from build123d import *

# Parameters (mm, degrees)
EXTRUDE_1_DEPTH     = 7.5
FILLET_1_R          = 3
FILLET_3_R          = 6
SKETCH_2_R          = 1.5
CUT_EXTRUDE_1_DEPTH = 10
SKETCH_5_R          = 4.5
EXTRUDE_2_DEPTH     = 15
SKETCH_4_R          = 1.5
CUT_EXTRUDE_3_DEPTH = 39.639358173
FILLET_2_R          = 6


with BuildPart() as part:
    # 草图1 → 凸台-拉伸1 (new, symmetric)
    with BuildSketch(Plane.XY):
        Polygon((-28, 5), (-28, 0), (-14, 0), (-14, 15), (0, 15), (0, 20), (-19, 20), (-19, 5), align=None)
        Polygon((0, 20), (0, 15), (14, 15), (14, 0), (28, 0), (28, 5), (19, 5), (19, 20), align=None)
    extrude(amount=EXTRUDE_1_DEPTH, both=True)

    # 圆角1
    fillet_1_edges = [part.edges().sort_by_distance(p)[0] for p in [
        (-19, 5, 0),
        (-19, 20, 0),
        (19, 20, 0),
        (19, 5, 0),
    ]]
    fillet(fillet_1_edges, radius=FILLET_1_R)

    # 圆角3
    fillet_3_edges = [part.edges().sort_by_distance(p)[0] for p in [
        (-14, 15, 0),
        (14, 15, 0),
    ]]
    fillet(fillet_3_edges, radius=FILLET_3_R)

    # 草图2 → 切除-拉伸1 (cut)
    with BuildSketch(Plane(origin=(0, 5, 0), x_dir=(1, 0, 0), z_dir=(0, 1, 0))):
        with Locations(Location((25, -4.5, 0), (0, 0, 180))):
            Circle(SKETCH_2_R)
        with Locations(Location((25, 4.5, 0), (0, 0, 180))):
            Circle(SKETCH_2_R)
    cut_extrude_1 = extrude(amount=-CUT_EXTRUDE_1_DEPTH, mode=Mode.SUBTRACT)

    # 草图5 → 凸台-拉伸2 (add)
    with BuildSketch(Plane.XY.offset(7.5)):
        with Locations((0, 17.5)):
            Circle(SKETCH_5_R)
    extrude(amount=-EXTRUDE_2_DEPTH)

    # 草图4 → 切除-拉伸3 (cut, through all)
    with BuildSketch(Plane.XY.offset(7.5)):
        with Locations((0, 17.5)):
            Circle(SKETCH_4_R)
    extrude(amount=-CUT_EXTRUDE_3_DEPTH, mode=Mode.SUBTRACT)

    # 镜向2: 切除-拉伸1 across plane
    add(cut_extrude_1.mirror(Plane(origin=(0, 0, 0), x_dir=(0, 0, 1), z_dir=(1, 0, 0))), mode=Mode.SUBTRACT)

    # 圆角2
    fillet_2_edges = [part.edges().sort_by_distance(p)[0] for p in [
        (-3.741657387, 15, 0),
        (-3.741657387, 20, 0),
        (3.741657387, 15, 0),
        (3.741657387, 20, 0),
    ]]
    fillet(fillet_2_edges, radius=FILLET_2_R)


solid = part.part
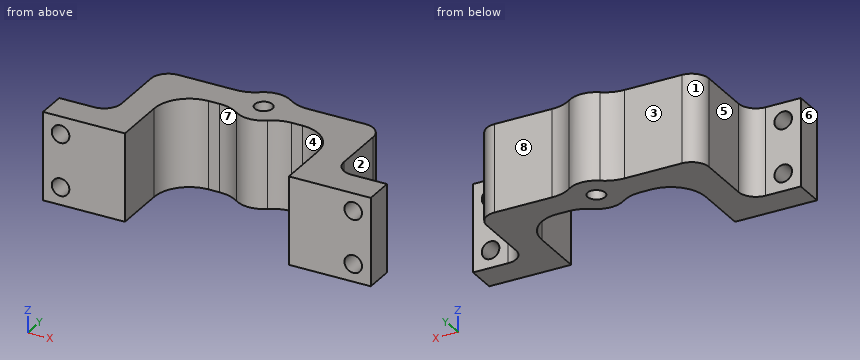
Could you check a few things on this model? Use its own coordinates, in mm. Face numbers are marked on the shaded views. A direction names the side the tool comes from. Give positions to 0.01 mm unless a question says otherwise; leave off trailing zeros. Write each loop counter-clockwise with the first axis right and the second up, starting at its lowest first coordinate (ties: lowest second). Pieces come first, ordered by that corner, then holes. Notation, with made-up numbers: (-19, 62) - (2, 62) arc R22 ccw to (2, 78) - close; hole circle Ø4 at (71.25, 81). An arc over 180 degrees is marked (long way). Use CSV: the item, a comma, the result in double quotes. Start each with the question number.
Item 1: I want a section at D-D, the plane z = 1.5. Please give me the cut outline in (x, y).
Item 2: If I drill on line 1 along Z through (x, y) = (-25, 1.75); line 2 along X through (y, z) = (2.75, -0.5); line 3 along X through (y, z) = (9, -3.75), over which ranges is the centre line in solid material (lowest first)?
Item 3: I want a section at C-C, the plane x = 0. Please give me the cut outline in (y, z), then the cut area to 3 significant figures.
Item 4: For the marked faces 5, 6, 7 and 8, which set-ups out of +Z, -Z, +X, -X, +Y, -Y let a thin tool reach every point of the face, with its end or its side?
Item 5: I'm going to push flat-ended pins straight in: pin 1 (2.5 mm diameter, centred on y = 12, z = -2.5, fed in from +X); pin 2 (0.6 mm diameter, centred on x = 7.5, z = -3.5, fed in from -Y); pin 3 (4 mm diameter, centred on x = -25, z = -4.5, fed in from -Y); pin 4 (6.5 mm diameter, centred on x = -26, z = -3.5, fed in from +Y). Where does each tip first touch, or does it pass through?
Item 6: I want a section at A-A, the plane y = 2.75. Please give me the cut outline in (x, z), then the cut area to 3 significant figures.
Item 7: If we mould it in two halves opening along X, with no side actions, what happens to the marked faces 1, 2, 3 and 4? For each: pulls with the +X half, pulls with the -X half, needs draft (parallel to the pull), parting line crosses it, or undercut.
Item 8: I want a section at B-B, the plane x = 25. Please give me the cut outline in (y, z), then the cut area to 3 significant figures.
Findings:
1,outline,"(-28, 0) - (-14, 0) - (-14, 9) arc R6 cw to (-8, 15) - (-6.16, 15) arc R6 cw to (-2.64, 13.86) arc R4.5 ccw to (2.64, 13.86) arc R6 cw to (6.16, 15) - (8, 15) arc R6 cw to (14, 9) - (14, 0) - (28, 0) - (28, 5) - (22, 5) arc R3 cw to (19, 8) - (19, 17) arc R3 ccw to (16, 20) - (6.16, 20) arc R6 cw to (2.64, 21.14) arc R4.5 ccw to (-2.64, 21.14) arc R6 cw to (-6.16, 20) - (-16, 20) arc R3 ccw to (-19, 17) - (-19, 8) arc R3 cw to (-22, 5) - (-28, 5) - close; hole circle Ø3 at (0, 17.5)"
2,line 1,"z = -7.5 to -6, -3 to 3, 6 to 7.5"
2,line 2,"x = -28 to -14, 14 to 28"
2,line 3,"x = -19 to -14, 14 to 19"
3,outline,"(13, -7.5) - (16, -7.5) - (16, 7.5) - (13, 7.5) - close; (19, -7.5) - (22, -7.5) - (22, 7.5) - (19, 7.5) - close"
3,area,"90.0 mm2"
4,face 5,"+Z, -Z, -X, +Y"
4,face 6,"+Z, -Z, -X, +Y, -Y"
4,face 7,"+Z, -Z, -Y"
4,face 8,"+Z, -Z, +X, +Y"
5,pin 1,"stops at x = 19"
5,pin 2,"stops at y = 15"
5,pin 3,"stops at y = 0"
5,pin 4,"stops at y = 5"
6,outline,"(-28, -7.5) - (-14, -7.5) - (-14, 7.5) - (-28, 7.5) - close; (14, -7.5) - (28, -7.5) - (28, 7.5) - (14, 7.5) - close; hole circle Ø3 at (-25, -4.5); hole circle Ø3 at (-25, 4.5); hole circle Ø3 at (25, -4.5); hole circle Ø3 at (25, 4.5)"
6,area,"392 mm2"
7,face 1,"pulls with the -X half"
7,face 2,"pulls with the +X half"
7,face 3,"needs draft"
7,face 4,"undercut"
8,outline,"(0, -7.5) - (5, -7.5) - (5, -6) - (0, -6) - close; (0, -3) - (5, -3) - (5, 3) - (0, 3) - close; (0, 6) - (5, 6) - (5, 7.5) - (0, 7.5) - close"
8,area,"45.0 mm2"
